```python
from build123d import *

# Parameters (mm, degrees)
SKETCH1_W      = 66.04
SKETCH1_H      = 68.58
EXTRUDE1_DEPTH = 20
FILLET1_R      = 5.08


with BuildPart() as part:
    # Sketch1 → Extrude1 (new body)
    with BuildSketch(Plane(origin=(0, 0, 0), x_dir=(1, 0, 0), z_dir=(0, 1, 0))):
        Rectangle(SKETCH1_W, SKETCH1_H)
    extrude(amount=EXTRUDE1_DEPTH)

    # Fillet1
    fillet1_edges = [part.edges().sort_by_distance(p)[0] for p in [
        (-33.02, 20, 0),
        (33.02, 20, 0),
        (-33.02, 0, 0),
        (33.02, 0, 0),
    ]]
    fillet(fillet1_edges, radius=FILLET1_R)


solid = part.part
```
Model file for the job. Use its own axes, mm. Coordinates: 2 decimals unless noted, no trailing zeros. Loops run counter-clockwise (first coordinate to the right, second up) from the corner with the lowest first, then second, coordinate; pieces in that order, holes last. Notation, with made-up numbers: (-28.75, 3.5) -> (-8.75, 3.5) arc R17 cw to (-8.75, 29.5) -> close; hole circle Ø1 at (78, 40). An arc over 180 degrees is marked (long way). Answer as a JSON object with one key per item and string values.
Q1. Flat gauge pin, fed straight in: P1, Ø4, axis at y = 2, z = -8, coming from the +X side. Where does the tip first touch, or does it go through?
Report:
{"P1": "stops at x = 32.9"}
Q2. Cut at A-A (z = 3). List the corners of the cut face in (x, y), and give its area (3 significant figures).
Report:
{"outline": "(-33.02, 5.08) arc R5.08 ccw to (-27.94, 0) -> (27.94, 0) arc R5.08 ccw to (33.02, 5.08) -> (33.02, 14.92) arc R5.08 ccw to (27.94, 20) -> (-27.94, 20) arc R5.08 ccw to (-33.02, 14.92) -> close", "area": "1,300 mm2"}
Q3. Cut at B-B (y = 2). List the corners of the cut face in (x, z), and give its area (3 significant figures).
Report:
{"outline": "(-31.98, -34.29) -> (31.98, -34.29) -> (31.98, 34.29) -> (-31.98, 34.29) -> close", "area": "4,390 mm2"}
Q4. Probe probe 1 along X at (y, z) = (15.75, -11.5); probe 2 along X at (y, z) = (17, -24); probe 3 along Y at (x, z) = (29.5, -0.5). List the from-to ranges inside material, lowest first.
Report:
{"probe 1": "x = -32.95 to 32.95", "probe 2": "x = -32.57 to 32.57", "probe 3": "y = 0.25 to 19.75"}
